The model under review builds one solid part; all positions refer to its coordinate system, in mm. Face numbers are marked on the shaded views. A direction names the side the tool comes from. Give positions to 0.01 mm unless a question says otherwise; leave off trailing zeros. Order: outer loops, then holes, each group sorted by start corner. A loop starts at its lowest first (then second) coordinate and runs counter-clockwise, first axis right, second up. Notation, with made-up numbers: (-13.5, 85) - (19.5, 85) arc R26 cw to (19.5, 121) - close; hole circle Ø5 at (75, 41). An arc over 180 degrees is marked (long way). Write item = value, one per line. Start each with the question number.
1. We need section B-B, the plane z = 0. Give the boundary of the cut face in (x, y), and give its area (3 significant figures).
2. Mouldability with a two-part tool opening along X and no side actions: class the marked faces 3, 4 and 5 as pulls with the +X half, pulls with the -X half, needs draft (parallel to the pull), parting line crosses it, or undercut.
3. We need section D-D, the plane x = -0.5. Give the boundary of the cut face in (y, z), and give its area (3 significant figures).
4. Wall thickness on probe 1 along X at (y, z) = (26, 1.5); probe 2 along Z at (x, y) = (14.15, 30); probe 3 along Z at (x, y) = (13.95, 18): over which ranges is each line inside the solid? List them lowest first.
5. We need section C-C, the plane y = 25.5. Give the boundary of the cut face in (x, z).
6. For P1, Ø1.5, axis at x = 2.5, z = -5, coming from the +Y side, flat-tipped, find the tip position at first contact; note if it passes through.
7. We need section A-A, the plane y = 30. Give the boundary of the cut face in (x, z), and give its area (3 significant figures).
8. Machinability: for the marked faces 1 and 2, which of the approach directions +Z, -Z, +X, -X, +Y, -Y give a long, thin tool a straight path to every point of the face, cutting with its end or side? Answer none if there is none.
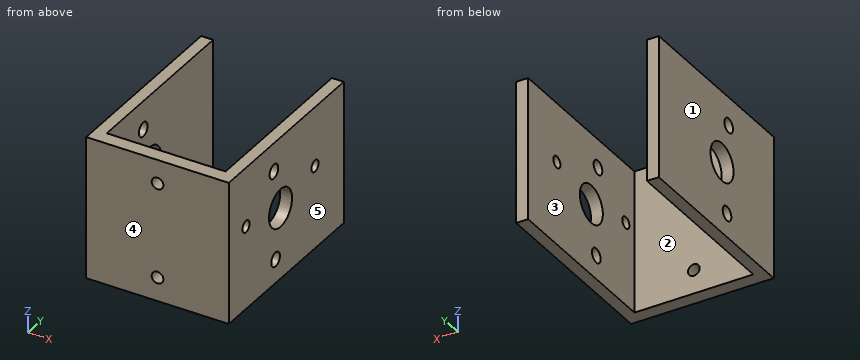
Autodesk Inventor part; units mm, degrees
ref_plane "作業平面1" through (0, 3, 15) normal (1, 0, 0) x (0, 0, -1)
ref_plane "YZ Plane" through (0, 0, 0) normal (1, 0, 0) x (0, 1, 0)
ref_plane "XZ Plane" through (0, 0, 0) normal (0, 1, 0) x (-1, 0, 0)
sketch "スケッチ1" plane through (0, 0, 0) normal (0, 1, 0) x (-1, 0, 0)
  line L0 (15, -15) -> (-15, -15)
  line L1 (-15, -15) -> (-15, 15)
  line L2 (-15, 15) -> (15, 15)
  line L3 (15, 15) -> (15, -15)
  line L4 (-15, 15) -> (15, -15) construction
  line L5 (-15, -15) -> (15, 15) construction
  point P0 (0, 0)
  point P1 (0, 0)
  dimension "d0" = 30
  dimension "d1" = 30
extrude "押し出し1" add sketch "スケッチ1" along normal blind 3
sketch "スケッチ2" plane through (0, 3, 0) normal (0, 1, 0) x (1, 0, 0)
  line L0 (-15, -15) -> (15, -15)
  line L1 (15, -15) -> (15, 15)
  line L2 (15, 15) -> (-15, 15)
  line L3 (-15, 15) -> (-15, -15)
  line L4 (-15, -15) -> (15, -15)
  line L5 (-15, -15) -> (-12.5, -15)
  line L6 (-12.5, -15) -> (-12.5, 15)
  line L7 (-12.5, 15) -> (-15, 15)
  line L8 (-15, 15) -> (-15, -15)
  line L9 (15, -15) -> (15, 15)
  line L10 (15, -15) -> (12.5, -15)
  line L11 (12.5, -15) -> (12.5, 15)
  line L12 (12.5, 15) -> (15, 15)
  line L13 (15, 15) -> (15, -15)
  line L14 (15, 15) -> (-15, 15)
  point P0 (0, 0)
  point P1 (-12.5, 15)
  dimension "d4" = 2.5
  dimension "d5" = 2.5
extrude "押し出し2" add sketch "スケッチ2" along normal blind 40 from surface at -3 contours L3 L2 L6 L0 | L11 L2 L1 L0
sketch "スケッチ3" plane through (15, 0, 15) normal (1, 0, 0) x (0, 0, -1)
  line L0 (0, 3) -> (30, 3)
  line L1 (15, 18) -> (30, 18) construction
  line L2 (30, 40) -> (30, 3) construction
  line L3 (15, 18) -> (-10.0782, 18) construction
  point P0 (15, 0)
  dimension "d8" = 15
  dimension "d50" = 15
hole "穴1" at (15, 18, 0) direction (-1, 0, 0) diameter 8 end through all
sketch "スケッチ6" plane through (0, 3, 0) normal (0, 1, 0) x (1, 0, 0)
  line L0 (12.5, 15) -> (-12.5, 15)
  point P0 (0, 0)
  point P1 (0, 10)
  point P2 (0, -10)
  point P3 (0, 15)
  dimension "d41" = 5
  dimension "d42" = 20
hole "穴3" at (0, 3, -10) at (0, 3, 10) direction (0, -1, 0) diameter 2.459 depth 3
sketch "スケッチ8" plane through (15, 0, 15) normal (1, 0, 0) x (0, 0, -1)
  circle A0 centre (15, 18) radius 4
  line L0 (12.5, 30) -> (12.5, 6) construction
  point P0 (15, 0)
  dimension "d56" = 24
  dimension "d57" = 12
  dimension "d58" = 2.5
hole "穴4" at (15, 30, 2.5) at (15, 6, 2.5) direction (-1, 0, 0) diameter 2.459 depth 2.5
sketch "スケッチ9" plane through (15, 0, 15) normal (1, 0, 0) x (0, 0, -1)
  circle A0 centre (15, 18) radius 4
  line L0 (0, 18) -> (15, 18)
  line L1 (0, 0) -> (0, 40)
  line L2 (30, 0) -> (30, 40)
  line L3 (15, 18) -> (-5.0402, 29.5702)
  line L4 (15, 18) -> (33.9658, 28.9499)
  circle A1 centre (6, 15.6906) radius 1.5
  circle A2 centre (25, 16.2679) radius 1.5
  line L5 (12.5, 13.6699) -> (-5.7345, 24.1976)
  line L6 (17.5, 13.6699) -> (25.6852, 18.3956)
  point P0 (15, 0)
  dimension "d70" = 3
  dimension "d71" = 3
  dimension "d72" = 6
  dimension "d73" = 5
  dimension "d83" = 5
  dimension "d84" = 5
  dimension "d85" = 30
  dimension "d86" = 30
hole "穴5" at (15, 15.6906, 9) at (15, 16.2679, -10) direction (-1, 0, 0) diameter 3 depth 30
ref_plane "作業平面1" through (0, 3, 15) normal (1, 0, 0) x (0, 0, -1)
properties part number "hand1" material "アルミニウム 6061"
Model answer:
q1.outline = (-15, 0) - (15, 0) - (15, 14) - (12.5, 14) - (12.5, 3) - (-12.5, 3) - (-12.5, 14) - (-15, 14) - close; (-15, 22) - (-12.5, 22) - (-12.5, 40) - (-15, 40) - close; (12.5, 22) - (15, 22) - (15, 40) - (12.5, 40) - close
q1.area = 235 mm2
q2.face_3 = undercut
q2.face_4 = needs draft
q2.face_5 = pulls with the +X half
q3.outline = (0, -15) - (3, -15) - (3, -11.12) - (0, -11.12) - close; (0, -8.88) - (3, -8.88) - (3, 8.88) - (0, 8.88) - close; (0, 11.12) - (3, 11.12) - (3, 15) - (0, 15) - close
q3.area = 76.5 mm2
q4.probe_1 = -15 to -12.5, 12.5 to 15
q4.probe_2 = -15 to 1.27, 3.73 to 15
q4.probe_3 = -15 to -4, 4 to 15
q5.outline = (-15, -15) - (-12.5, -15) - (-12.5, 15) - (-15, 15) - close; (12.5, -15) - (15, -15) - (15, 15) - (12.5, 15) - close
q6.P1 = 3
q7.outline = (-15, -15) - (-12.5, -15) - (-12.5, 15) - (-15, 15) - close; (12.5, -15) - (15, -15) - (15, 1.27) - (12.5, 1.27) - close; (12.5, 3.73) - (15, 3.73) - (15, 15) - (12.5, 15) - close
q7.area = 144 mm2
q8.face_1 = +Z, -Z, -X, +Y, -Y
q8.face_2 = +Z, -Z, +Y
